from build123d import *

# Parameters (mm, degrees)
F1_DEPTH  = 13
F2_W      = 10
F2_H      = 7
F3_DEPTH  = 6.001
F5_DEPTH  = 13.001
F6_R      = 1.25
F7_DEPTH  = 6.001
F8_R      = 1.25
F8_W      = 5
F8_H      = 19
F9_DEPTH  = 6
F10_R     = 1.65
F11_DEPTH = 27.001
F12_W     = 5
F12_H     = 19
F12_R     = 1.25
F13_DEPTH = 6
F14_R     = 1.65
F15_DEPTH = 27.001


with BuildPart() as f1:
    # F0 (on Top) → F1 (new body)
    with BuildSketch(Plane.XY):
        Polygon((38.8, 3), (-33.8, 3), (-33.8, -3), (-6, -3), (6, -3), (38.8, -3), align=None)
    extrude(amount=F1_DEPTH)

    # F2 (on face) → F3 (cut, through all)
    with BuildSketch(Plane(origin=(0, 3, 0), x_dir=(-1, 0, 0), z_dir=(0, 1, 0))):
        Polygon((-28.8, 7), (-28.8, 0), (-21.8, 0), align=None)
        with Locations((-33.8, 3.5)):
            Rectangle(F2_W, F2_H)
        Polygon((20.5147186258, 13), (-25.5147186258, 13), (-19.3147186258, 6), (14.3147186258, 6), align=None)
        Polygon((23.8, 7), (16.8, 0), (23.8, 0), align=None)
        with Locations((28.8, 3.5)):
            Rectangle(F2_W, F2_H)
    extrude(amount=-F3_DEPTH, mode=Mode.SUBTRACT)

    # F4 (on face) → F5 (cut, through all)
    with BuildSketch(Plane(origin=(0, 0, 0), x_dir=(1, 0, 0), z_dir=(0, 0, -1))):
        with BuildLine():
            Line((-6, -3), (6, -3))
            ThreePointArc((6, -3), (0, -0.7), (-6, -3))
        make_face()
    extrude(amount=-F5_DEPTH, mode=Mode.SUBTRACT)

    # F6 (on face) → F7 (cut, through all)
    with BuildSketch(Plane.XZ.offset(3)):
        with Locations((-1.8, 3)):
            Circle(F6_R)
        with Locations((6.8, 3)):
            Circle(F6_R)
    extrude(amount=-F7_DEPTH, mode=Mode.SUBTRACT)

    # F8 (on face) → F9 (join)
    with BuildSketch(Plane.YZ.offset(38.8)):
        with BuildLine():
            Line((3, 13), (3, 7))
            Line((3, 7), (17.3542486889, 7))
            ThreePointArc((17.3542486889, 7), (24, 10), (17.3542486889, 13))
            Line((17.3542486889, 13), (3, 13))
        make_face()
        with Locations((20, 10)):
            Circle(F8_R, mode=Mode.SUBTRACT)
        with Locations((-0.5, 22.5)):
            Rectangle(F8_W, F8_H)
        Polygon((-3, 13), (-3, 7), (3, 7), (3, 13), (2, 13), align=None)
    extrude(amount=F9_DEPTH)

    # F10 (on face) → F11 (cut, through all)
    with BuildSketch(Plane.XZ.offset(3)):
        with Locations((41.8, 16.4)):
            Circle(F10_R)
        with Locations((41.8, 28.4)):
            Circle(F10_R)
    extrude(amount=-F11_DEPTH, mode=Mode.SUBTRACT)

    # F12 (on face) → F13 (join)
    with BuildSketch(Plane(origin=(-33.8, 0, 0), x_dir=(0, -1, 0), z_dir=(-1, 0, 0))):
        with Locations((0.5, 22.5)):
            Rectangle(F12_W, F12_H)
        with BuildLine():
            Line((-17.3542486889, 7), (-3, 7))
            Line((-3, 7), (-3, 13))
            Line((-3, 13), (-17.3542486889, 13))
            ThreePointArc((-17.3542486889, 13), (-24, 10), (-17.3542486889, 7))
        make_face()
        with Locations((-20, 10)):
            Circle(F12_R, mode=Mode.SUBTRACT)
        Polygon((3, 7), (3, 13), (-2, 13), (-3, 13), (-3, 7), align=None)
    extrude(amount=F13_DEPTH)

    # F14 (on face) → F15 (cut, through all)
    with BuildSketch(Plane.XZ.offset(3)):
        with Locations((-36.8, 28.4)):
            Circle(F14_R)
        with Locations((-36.8, 16.4)):
            Circle(F14_R)
    extrude(amount=-F15_DEPTH, mode=Mode.SUBTRACT)


solid = f1.part
Work out the finished part from the listing and answer in its coordinate system (mm). A direction names the side the tool comes from. Round coordinates to 2 decimals unless told otherwise and drop trailing zeros. Write each loop counter-clockwise with the first axis right and the second up, starting at its lowest first coordinate (ties: lowest second). Pieces come first, ordered by that corner, then holes. Notation, with made-up numbers: M 47,-13.5 L 87,-13.5 A19 cw 87,8.5 Z; hole C 88,70 d9. An arc over 180 degrees is marked long. Use a Markdown table: item, result.
1) Consider line 1 (Z direction, x = -36.8, y = 0.5); line 2 (Z direction, x = -1.8, y = -1.5); line 3 (X direction, y = 9.5, z = 11). Determine where each line is inside the solid, lowest interval first. Write a range as [from, to].
Taken from the geometry:
| item | result |
|---|---|
| line 1 | z = [7, 14.75], [18.05, 26.75], [30.05, 32] |
| line 2 | z = [0, 1.75], [4.25, 6] |
| line 3 | x = [-39.8, -33.8], [38.8, 44.8] |
2) Determine the mould class of faces 4 (the face through (-3.05, -0.91, 3.05)), 5 (the face through (-36.758, 19.328, 11.054)), 6 (the face through (22.46, 0.04, 9.55)), 7 (the face through (-20.3, 0, 3.5)) for opening direction Z: pulls with the +Z half, pulls with the -Z half, needs draft (parallel to the pull), parting line crosses it, or undercut.
Taken from the geometry:
| item | result |
|---|---|
| face 4 | undercut |
| face 5 | undercut |
| face 6 | pulls with the +Z half |
| face 7 | pulls with the -Z half |
3) Which of the six approach directions +Z, -Z, +X, -X, +Y, -Y give full straight-line access (tool end or side, diameter ignored) to faces 1 (the face through (3, 0, 6)), 2 (the face through (42, 2, 22)), 3 (the face through (-20, 3, 6))?
Taken from the geometry:
| item | result |
|---|---|
| face 1 | +Z, +Y, -Y |
| face 2 | +Z, +X, -X |
| face 3 | +Z, -Z, +Y |
4) The part is cut by section B-B on y = 14.25. Give the vertices of the cut face in (x, z).
Taken from the geometry:
| item | result |
|---|---|
| outline | M -39.8,7 L -33.8,7 L -33.8,13 L -39.8,13 Z; M 38.8,7 L 44.8,7 L 44.8,13 L 38.8,13 Z |
5) The part is cut by section C-C on z = 28.4. Give the vertices of the cut face in (x, y), plus the area to 3 significant figures.
Taken from the geometry:
| item | result |
|---|---|
| outline | M -39.8,-3 L -38.45,-3 L -38.45,2 L -39.8,2 Z; M -35.15,-3 L -33.8,-3 L -33.8,2 L -35.15,2 Z; M 38.8,-3 L 40.15,-3 L 40.15,2 L 38.8,2 Z; M 43.45,-3 L 44.8,-3 L 44.8,2 L 43.45,2 Z |
| area | 27.0 mm2 |
6) The part is cut by section A-A on x = 41.8. Give the vertices of the cut face in (y, z), plus the area to 3 significant figures.
Taken from the geometry:
| item | result |
|---|---|
| outline | M -3,7 L 17.35,7 A4 ccw long 17.35,13 L 2,13 L 2,14.75 L -3,14.75 Z; M -3,18.05 L 2,18.05 L 2,26.75 L -3,26.75 Z; M -3,30.05 L 2,30.05 L 2,32 L -3,32 Z; hole C 20,10 d2.5 |
| area | 224 mm2 |
7) The part is cut by section D-D on x = 6.8. Give the vertices of the cut face in (y, z).
Taken from the geometry:
| item | result |
|---|---|
| outline | M -3,0 L 3,0 L 3,1.75 L -3,1.75 Z; M -3,4.25 L 3,4.25 L 3,6 L -3,6 Z |
8) Flat-ended cylindrical pins translate along their axes: pin 1 (4 mm diameter, centred on x = -1.8, z = 3, fed in from +Y); pin 2 (3 mm diameter, centred on x = 28.5, y = 2.5, fed in from -Z); pin 3 (13 mm diameter, centred on x = -31, y = 12, fed in from -Z). Find the tip coordinate at first contact, or state that the pin passes through.
Taken from the geometry:
| item | result |
|---|---|
| pin 1 | stops at y = 1.54 |
| pin 2 | stops at z = 5.2 |
| pin 3 | stops at z = 6.62 |
